The listing builds one solid part. Answer for the finished solid, in the listing's coordinates (mm). A direction names the side the tool comes from. Give positions to 0.01 mm unless a question says otherwise; leave off trailing zeros. Write each loop counter-clockwise with the first axis right and the second up, starting at its lowest first coordinate (ties: lowest second). Pieces come first, ordered by that corner, then holes. Notation, with made-up numbers: (53, 75.5) - (96, 75.5) arc R14 ccw to (96, 93.5) - close; hole circle Ø11 at (28.25, 13.5). An arc over 180 degrees is marked (long way). Answer as CSV lines item,"result". Start each with the question number.
(1) Find section B-B (z = -8.5). Write down the section's boundary in (x, y), then the cut area to 3 significant figures.
(2) For faces 5 (the face through (40, -40, 0)), 6 (the face through (2.46, -6.79, -6.9)), determine the directions among +Z, -Z, +X, -X, +Y, -Y from which every point of the face is accessible in a straight line to the end or side of a thin tool.
(3) Straight lines are drawn through the part: probe 1 along Y at (x, z) = (1.15, 0); probe 2 along X at (y, z) = (-15.5, 2.5); probe 3 along Y at (x, z) = (50.5, 6). For each, find the intervals that lie inside material, in ascending order.
(4) Find section D-D (z = 16). Write down the section's boundary in (x, y), then the cut area to 3 significant figures.
(5) Each of these flat-tipped pins is pushed along its axis until it touches: pin 1 Ø2.5 at (y, z) = (-5.88, -8.09) entering from -X; pin 2 Ø12 at (y, z) = (9, -7.5) entering from +X; pin 3 Ø12 at (x, z) = (16.5, -11) entering from +Y; pin 4 Ø3 at (y, z) = (-37.5, 7.5) entering from +X. Where does it stop, or does it pass through?
(6) Find section A-A (z = 0). Write down the section's boundary in (x, y).
(7) For a pull along Y with two mould halves and no side action, classify faces 1 (the face through (2.46, 0.07, 11.5)), 2 (the face through (5, -4, 0)), 3 (the face through (2, 20, 0)), 4 (the face through (27, -50, 0)) as pulls with the +Y half, pulls with the -Y half, needs draft (parallel to the pull), parting line crosses it, or undercut.
(8) Find section C-C (x = 16.5). Write down the section's boundary in (y, z).
from build123d import *

# Parameters (mm, degrees)
SKETCH1_R            = 1.5
SKETCH1_R_2          = 2.5
BOSS_EXTRUDE11_DEPTH = 5
SKETCH2_W            = 40
SKETCH2_H            = 10
BOSS_EXTRUDE12_DEPTH = 50
CHAMFER1_SIZE        = 20


with BuildPart() as part:
    # Sketch1 → Boss-Extrude11 (new body)
    with BuildSketch(Plane(origin=(0, 0, 0), x_dir=(0, 0, -1), z_dir=(1, 0, 0))):
        with BuildLine():
            Line((-20, 0), (-20, -50))
            Line((-20, -50), (20, -50))
            Line((20, -50), (20, 0))
            ThreePointArc((20, 0), (0, 20), (-20, 0))
        make_face()
        with Locations((-10, 0)):
            Circle(SKETCH1_R, mode=Mode.SUBTRACT)
        Circle(SKETCH1_R_2, mode=Mode.SUBTRACT)
        with Locations((8.090169944, -5.877852523)):
            Circle(SKETCH1_R, mode=Mode.SUBTRACT)
        with Locations((-3.090169944, -9.510565163)):
            Circle(SKETCH1_R, mode=Mode.SUBTRACT)
        with Locations((8.090169944, 5.877852523)):
            Circle(SKETCH1_R, mode=Mode.SUBTRACT)
        with Locations((-3.090169944, 9.510565163)):
            Circle(SKETCH1_R, mode=Mode.SUBTRACT)
    extrude(amount=BOSS_EXTRUDE11_DEPTH)

    # Sketch2 → Boss-Extrude12 (add)
    with BuildSketch(Plane(origin=(5, 0, 0), x_dir=(0, 0, -1), z_dir=(1, 0, 0))):
        with Locations((0, -45)):
            Rectangle(SKETCH2_W, SKETCH2_H)
    extrude(amount=BOSS_EXTRUDE12_DEPTH)

    # Chamfer1
    chamfer1_edges = [part.edges().sort_by_distance(p)[0] for p in [
        (5, -40, 0),
    ]]
    chamfer(chamfer1_edges, length=CHAMFER1_SIZE)


solid = part.part
Result set:
1,outline,"(0, -50) - (55, -50) - (55, -40) - (25, -40) - (5, -20) - (5, -7.32) - (0, -7.32) - close; (0, -4.43) - (5, -4.43) - (5, 4.43) - (0, 4.43) - close; (0, 7.32) - (5, 7.32) - (5, 18.1) - (0, 18.1) - close"
1,area,"1,010 mm^2"
2,face 5,"+Z, -Z, +X, +Y"
2,face 6,"+X, -X"
3,probe 1,"-50 to -2.5, 2.5 to 20"
3,probe 2,"0 to 5"
3,probe 3,"-50 to -40"
4,outline,"(0, -50) - (55, -50) - (55, -40) - (25, -40) - (5, -20) - (5, 12) - (0, 12) - close"
4,area,"1,010 mm^2"
5,pin 1,"through"
5,pin 2,"x = 5"
5,pin 3,"y = -25.5"
5,pin 4,"x = 24"
6,outline,"(0, -50) - (55, -50) - (55, -40) - (25, -40) - (5, -20) - (5, -2.5) - (0, -2.5) - close; (0, 2.5) - (5, 2.5) - (5, 20) - (0, 20) - close"
7,face 1,"undercut"
7,face 2,"needs draft"
7,face 3,"pulls with the +Y half"
7,face 4,"pulls with the -Y half"
8,outline,"(-50, -20) - (-31.5, -20) - (-31.5, 20) - (-50, 20) - close"
